Part model, mm, in its own coordinate system. A direction names the side the tool comes from. Give positions to 0.01 mm unless a question says otherwise; leave off trailing zeros. Write each loop counter-clockwise with the first axis right and the second up, starting at its lowest first coordinate (ties: lowest second). Pieces come first, ordered by that corner, then holes.
from build123d import *

# Parameters (mm, degrees)
BOSS_EXTRUDE1_DEPTH = 4.5


with BuildPart() as part:
    # Sketch1 → Boss-Extrude1 (new body)
    with BuildSketch(Plane(origin=(0, 0, 0), x_dir=(1, 0, 0), z_dir=(0, 1, 0))):
        Polygon((-30.066262521, 37.5), (-40, 37.5), (-40, 30), (-48, 30), (-48, 15), (-40, 15), (-40, 12.5), (-40, -15), (-48, -15), (-48, -30), (-40, -30), (-40, -32.5), (-40, -34.271597524), (-40, -37.5), (40, -37.5), (40, -32.5), (40, -30), (48, -30), (48, -17.5), (48, -15), (40, -15), (40, 12.5), (40, 15), (48, 15), (48, 30), (40.57, 30), (40.57, 37.5), (30.636262521, 37.5), (30.636262521, 45.5), (10.636262521, 45.5), (10.636262521, 37.5), (-9.496262521, 37.5), (-9.496262521, 45.5), (-30.066262521, 45.5), align=None)
    extrude(amount=-BOSS_EXTRUDE1_DEPTH)


solid = part.part
1) Saw through at C-C (z = -8). Write the cut outline in (x, y).
Check result:
outline: (-40, -4.5) - (40, -4.5) - (40, 0) - (-40, 0) - close
2) Saw through at D-D (x = -35.5). Write the cut outline in (y, z).
Check result:
outline: (-4.5, -37.5) - (0, -37.5) - (0, 37.5) - (-4.5, 37.5) - close
3) Drill centre lines: L1, parallel to Z at x = -42, y = -2.15; L2, parallel to X at y = -1.1, z = -40; L3, parallel to Z at x = 4, y = -2.55. Where is each one in solid material? Low to high.
Check result:
L1: z = -30 to -15, 15 to 30
L2: x = -30.07 to -9.5, 10.64 to 30.64
L3: z = -37.5 to 37.5
4) Saw through at B-B (y = -1.1). Write the cut outline in (x, z).
Check result:
outline: (-48, -30) - (-40, -30) - (-40, -37.5) - (-30.07, -37.5) - (-30.07, -45.5) - (-9.5, -45.5) - (-9.5, -37.5) - (10.64, -37.5) - (10.64, -45.5) - (30.64, -45.5) - (30.64, -37.5) - (40.57, -37.5) - (40.57, -30) - (48, -30) - (48, -15) - (40, -15) - (40, 15) - (48, 15) - (48, 30) - (40, 30) - (40, 37.5) - (-40, 37.5) - (-40, 30) - (-48, 30) - (-48, 15) - (-40, 15) - (-40, -15) - (-48, -15) - close
5) 3-axis set-ups, long thin cutter, end or side, ignore diameter. For faces 4 (the flat face through (-40, -2, 0)), 5 (the flat face through (-9.496, -2, -41)), 6 (the flat face through (-40, -2, 34)), 7 (the flat face through (44, -2, -30)): which of +Z, -Z, +X, -X, +Y, -Y reach the whole face in a straight line?
Check result:
face 4: -X, +Y, -Y
face 5: -Z, +Y, -Y
face 6: +Z, -X, +Y, -Y
face 7: -Z, +X, +Y, -Y
6) Saw through at A-A (x = 42). Write the cut outline in (y, z), and give its area (3 significant figures).
Check result:
outline: (-4.5, -30) - (0, -30) - (0, -15) - (-4.5, -15) - close; (-4.5, 15) - (0, 15) - (0, 30) - (-4.5, 30) - close
area: 135 mm2
7) Mould opens along Z. For faces 1 (the flat face through (44, -2, -15)), 2 (the flat face through (48, -2, 23)), 3 (the flat face through (44, -2, 30)) say: +Z half, -Z half, draft (parallel to the pull), parting line (faces both ways), or undercut.
Check result:
face 1: undercut
face 2: draft
face 3: +Z half
8) Flat gauge pins, fed straight in: P1, Ø1.3, axis at y = -2, z = 7, coming from the +X side; P2, Ø1.5, axis at y = -2, z = -13.5, coming from the -X side; P3, Ø1.3, axis at x = -45, y = -3, coming from the -Z side. Where does each tip first touch, or does it go through?
Check result:
P1: stops at x = 40
P2: stops at x = -40
P3: stops at z = -30
